Could you check a few things on this model? Use its own coordinates, in mm. Face numbers are marked on the shaded views. A direction names the side the tool comes from. Round coordinates to 2 decimals unless told otherwise and drop trailing zeros. Loops run counter-clockwise (first coordinate to the right, second up) from the corner with the lowest first, then second, coordinate; pieces in that order, holes last. Notation, with made-up numbers: (-6, 33) -> (8, 33) arc R6 cw to (8, 43) -> close; hole circle Ø5 at (30, 24). An arc over 180 degrees is marked (long way). One line per item, written item: value.
Autodesk Inventor part; units mm, degrees
ref_plane "YZ Plane" through (0, 0, 0) normal (1, 0, 0) x (0, 1, 0)
ref_plane "XZ Plane" through (0, 0, 0) normal (0, 1, 0) x (-1, 0, 0)
ref_plane "XY Plane" through (0, 0, 0) normal (0, 0, 1) x (1, 0, 0)
sketch "Sketch1" plane through (0, 0, 0) normal (0, 1, 0) x (-1, 0, 0)
  line L0 (0, 0) -> (90, 0)
  line L1 (90, 0) -> (90, -70)
  line L2 (90, -70) -> (0, -70)
  circle A0 centre (85, -65) radius 1.6095
  circle A1 centre (85, -5) radius 1.6095
  circle A2 centre (5, -65) radius 1.6095
  circle A3 centre (5, -5) radius 1.6095
  line L3 (11.9037, -61.65) -> (11.9037, -67.5)
  line L4 (11.9037, -67.5) -> (77.409, -67.5)
  line L5 (77.409, -67.5) -> (77.409, -58.5)
  line L6 (87.5, -35) -> (87.5, -58.5)
  line L7 (87.5, -58.5) -> (77.409, -58.5)
  line L8 (11.9037, -61.65) -> (0, -61.65)
  line L9 (0, -61.65) -> (0, -70)
  line L10 (11.9037, -8.35) -> (11.9037, -2.5)
  line L11 (11.9037, -2.5) -> (77.409, -2.5)
  line L12 (77.409, -2.5) -> (77.409, -11.5)
  line L13 (87.5, -35) -> (87.5, -11.5)
  line L14 (87.5, -11.5) -> (77.409, -11.5)
  line L15 (11.9037, -8.35) -> (0, -8.35)
  line L16 (0, -8.35) -> (0, 0)
  line L17 (99.038, -35) -> (-9.0118, -35) construction
  point P0 (11.9037, -5.425)
  dimension "d34" = 70
  dimension "d35" = 60
  dimension "d37" = 10.091
  dimension "d38" = 65.5053
  dimension "d39" = 60
  dimension "d40" = 70
  dimension "d41" = 9
  dimension "d43" = 90
  dimension "d44" = 11.9037
  dimension "d45" = 3.219
  dimension "d46" = 47
  dimension "d47" = 5.85
  dimension "d48" = 8.35
  dimension "d49" = 5
  dimension "d50" = 5
  dimension "d51" = 5
  dimension "d52" = 5
extrude "Extrusion1" add sketch "Sketch1" along normal blind 20 contours L0 L1 L2 L9 L8 L3 L4 L5 L7 L6 L13 L14 L12 L11 L10 L15 L16 | A0 | A1 | A2 | A3
sketch "Sketch2" plane through (0, 20, 0) normal (0, 1, 0) x (1, 0, 0)
  line L0 (0, 70) -> (-90, 70)
  circle A0 centre (-4.9798, 65) radius 1.6095
  line L1 (-90, 70) -> (-90, 0)
  circle A1 centre (-85.0202, 65) radius 1.6095
  circle A2 centre (-4.9798, 5) radius 1.6095
  circle A3 centre (-85.0202, 5) radius 1.6095
  point P0 (0, 0)
extrude "Extrusion2" cut sketch "Sketch2" against normal blind 30
fillet "Fillet1" radius 7 4 edges at (-90, 10, 0) (-90, 10, -70) (0, 10, -70) (0, 10, 0)
sketch "Sketch4" plane through (0, 20, 0) normal (0, 1, 0) x (1, 0, 0)
  line L0 (-77.409, 11.5) -> (-77.409, 58.5)
  line L1 (-77.409, 58.5) -> (-87.5, 58.5)
  line L2 (-87.5, 58.5) -> (-87.5, 11.5)
  line L3 (-87.5, 11.5) -> (-77.409, 11.5)
  point P0 (0, 0)
extrude "Extrusion3" add sketch "Sketch4" against normal blind 2
sketch "Sketch5" plane through (0, 20, 0) normal (0, 1, 0) x (1, 0, 0)
  line L0 (-11.9037, 61.65) -> (-11.9037, 8.35)
  line L1 (-11.9037, 8.35) -> (0, 8.35)
  line L2 (0, 8.35) -> (0, 61.65)
  line L3 (0, 61.65) -> (-11.9037, 61.65)
  line L4 (-11.9037, 61.65) -> (-77.409, 61.65)
  line L5 (-77.409, 58.5) -> (-77.409, 67.5)
  line L6 (-77.409, 67.5) -> (-77.409, 61.65)
  line L7 (-11.9037, 61.65) -> (-11.9037, 67.5)
  line L8 (-11.9037, 67.5) -> (-77.409, 67.5)
  line L9 (-11.9037, 2.5) -> (-77.409, 2.5)
  line L10 (-11.9037, 8.35) -> (-11.9037, 2.5)
  line L11 (-11.9037, 2.5) -> (-77.409, 2.5)
  line L12 (-77.409, 2.5) -> (-77.409, 8.35)
  line L13 (-77.409, 8.35) -> (-11.9037, 8.35)
  point P0 (0, 0)
extrude "Extrusion4" add sketch "Sketch5" against normal blind 2
fillet "Fillet2" radius 5 1 edges at (-77.409, 9, -58.5)
fillet "Fillet3" radius 5 1 edges at (-77.409, 9, -11.5)
fillet "Fillet4" radius 5 4 edges at (-77.409, 19, -61.65) (-11.9037, 19, -61.65) (-11.9037, 19, -8.35) (-77.409, 19, -8.35)
sketch "Sketch6" plane through (0, 20, 0) normal (0, 1, 0) x (1, 0, 0)
  line L0 (-77.409, 67.5) -> (-11.9037, 67.5)
  line L1 (-11.9037, 67.5) -> (-11.9037, 2.5)
  line L2 (-11.9037, 2.5) -> (-77.409, 2.5)
  line L3 (-77.409, 2.5) -> (-77.409, 67.5)
  point P0 (0, 0)
extrude "Extrusion5" cut sketch "Sketch6" against normal blind 10
properties part number "Módulo de fixação Eletrônicos" material "PPS Plastic"
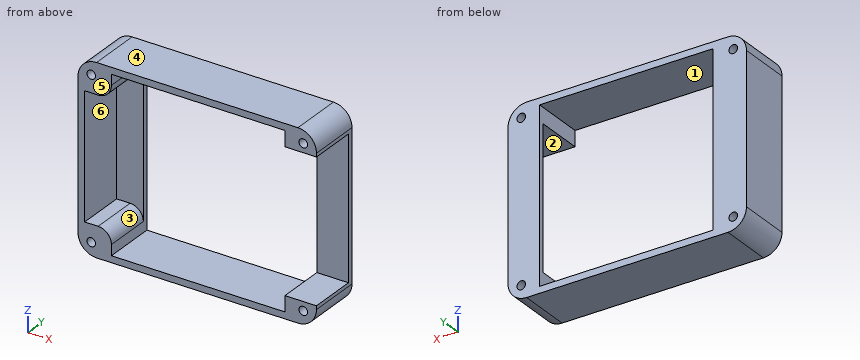
(1) Imagine slicing it at A-A on z = -57. Write out the boundary of the cut face in (x, y), then the cut area to 3 significant figures.
Results below:
outline: (-90, 0) -> (-87.5, 0) -> (-87.5, 18) -> (-77.41, 18) -> (-77.41, 20) -> (-90, 20) -> close; (-11.9, 18) -> (0, 18) -> (0, 20) -> (-11.9, 20) -> close
area: 94.0 mm²
(2) For pin 1 Ø1.5 at (x, y) = (-85.5, 5.5) entering from -Z; pin 2 Ø2.5 at (x, y) = (-85, 10) entering from +Z; pin 3 Ø3 at (x, z) = (-82, -25.5) entering from -Y, each with a flat end and sliding along its axis, tell me the tip position at first contact or that it passes through.
Results below:
pin 1: stops at z = -69.78
pin 2: stops at z = -0.04
pin 3: stops at y = 18
(3) Imagine slicing it at C-C on x = -33. Write out the boundary of the cut face in (y, z).
Results below:
outline: (0, -70) -> (20, -70) -> (20, -67.5) -> (0, -67.5) -> close; (0, -2.5) -> (20, -2.5) -> (20, 0) -> (0, 0) -> close
(4) We'd pull the mould along Z, two halves only. Please class the marked faces 4, 5 and 6: +Z half, -Z half, draft (parallel to the pull), parting line (faces both ways), or undercut.
Results below:
face 4: +Z half
face 5: draft
face 6: undercut
(5) On a 3-axis mill with a long thin cutter (end or side, diameter ignored), from which of +Z, -Z, +X, -X, +Y, -Y can I reach the whole of each face in a straight line? I mean the marked faces 1, 2 and 3. Say none if no direction works.
Results below:
face 1: +Y, -Y
face 2: +X, -Y
face 3: -Y
(6) Imagine slicing it at D-D on z = -65. Write out the boundary of the cut face in (x, y).
Results below:
outline: (-89.71, 0) -> (-86.63, 0) -> (-86.63, 20) -> (-89.71, 20) -> close; (-83.41, 0) -> (-77.41, 0) -> (-77.41, 20) -> (-83.41, 20) -> close; (-11.9, 0) -> (-6.59, 0) -> (-6.59, 20) -> (-11.9, 20) -> close; (-3.37, 0) -> (-0.29, 0) -> (-0.29, 20) -> (-3.37, 20) -> close
(7) Imagine slicing it at B-B on y = 9. Write out the boundary of the cut face in (x, z).
Results below:
outline: (-90, -63) arc R7 ccw to (-83, -70) -> (-7, -70) arc R7 ccw to (0, -63) -> (0, -61.65) -> (-11.9, -61.65) -> (-11.9, -67.5) -> (-77.41, -67.5) -> (-77.41, -63.5) arc R5 ccw to (-82.41, -58.5) -> (-87.5, -58.5) -> (-87.5, -11.5) -> (-82.41, -11.5) arc R5 ccw to (-77.41, -6.5) -> (-77.41, -2.5) -> (-11.9, -2.5) -> (-11.9, -8.35) -> (0, -8.35) -> (0, -7) arc R7 ccw to (-7, 0) -> (-83, 0) arc R7 ccw to (-90, -7) -> close; hole circle Ø3.22 at (-85.02, -65); hole circle Ø3.22 at (-85.02, -5); hole circle Ø3.22 at (-4.98, -65); hole circle Ø3.22 at (-4.98, -5)
(8) Please list where these lines run through material, in increasing order: L1, parallel to X at y = 6, z = -65; L2, parallel to Z at x = -73.5, y = 3.5; L3, parallel to Z at x = -7, y = 7.5.
Results below:
L1: x = -89.71 to -86.63, -83.41 to -77.41, -11.9 to -6.59, -3.37 to -0.29
L2: z = -70 to -67.5, -2.5 to 0
L3: z = -70 to -61.65, -8.35 to 0
